```python
from build123d import *

# Parameters (mm, degrees)
SKETCH1_W      = 25.4
SKETCH1_H      = 12.7
SKETCH1_R      = 1.27
EXTRUDE1_DEPTH = 7.62
CHAMFER1_SIZE  = 1.27


with BuildPart() as part:
    # Sketch1 → Extrude1 (new body)
    with BuildSketch(Plane.XY):
        with Locations((12.7, 6.35)):
            Rectangle(SKETCH1_W, SKETCH1_H)
        with Locations((16.51, 6.35)):
            Circle(SKETCH1_R, mode=Mode.SUBTRACT)
    extrude(amount=EXTRUDE1_DEPTH)

    # Chamfer1
    chamfer1_edges = [part.edges().sort_by_distance(p)[0] for p in [
        (0, 6.35, 7.62),
        (0, 6.35, 0),
        (0, 12.7, 3.81),
        (25.4, 12.7, 3.81),
        (25.4, 0, 3.81),
        (0, 0, 3.81),
    ]]
    chamfer(chamfer1_edges, length=CHAMFER1_SIZE)

    # Sketch2 → CBORE for #8 Socket Head Cap Screw1 (revolve, cut)
    with BuildSketch(Plane(origin=(16.51, 6.35, 7.62), x_dir=(0, -1, 0), z_dir=(1, 0, 0))):
        Polygon((0, 0), (0, 7.62), (2.8829, 7.62), (2.2479, 6.985), (2.2479, 4.8006), (2.8829, 4.1656), (3.96875, 4.1656), (3.96875, 0.635), (4.60375, 0), align=None)
    revolve(axis=Axis((16.51, 6.35, 13.97), (0, 0, -1)), mode=Mode.SUBTRACT)

    # Sketch4 → CBORE for #4 Socket Head Cap Screw1 (revolve, cut)
    with BuildSketch(Plane(origin=(3.81, 6.35, 0), x_dir=(0, 1, 0), z_dir=(1, 0, 0))):
        Polygon((0, 0), (0, 7.62), (1.5875, 7.62), (1.5875, 1.524), (1.6002, 1.524), (1.6002, 0.3048), (1.905, 0), align=None)
    revolve(axis=Axis((3.81, 6.35, -6.35), (0, 0, 1)), mode=Mode.SUBTRACT)


solid = part.part
```
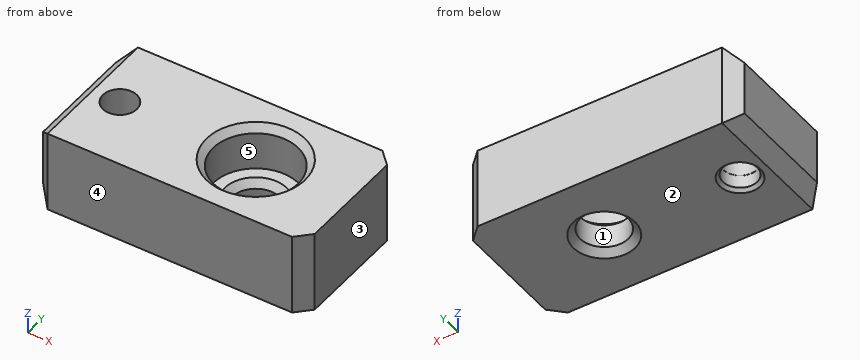
Source: CAD feature listing. Evaluate the final solid. Frame: model axes, mm. Face numbers are marked on the shaded views. A direction names the side the tool comes from. Give positions to 0.01 mm unless a question says otherwise; leave off trailing zeros. Order: outer loops, then holes, each group sorted by start corner. A loop starts at its lowest first (then second) coordinate and runs counter-clockwise, first axis right, second up.
(1) Material intervals for line 1 along X through (y, z) = (6.35, 4.9); line 2 along X through (y, z) = (6.35, 2.1); line 3 along Y through (x, z) = (3.81, 5), sorted ascending.
(2) Section query A-A (y = 6.35). State how many separate pieces and enclosed holes the cut face has, plus the area to 3 significant figures.
(3) Contact query for flat-ended pins moving along their axis: P1, Ø5, axis at x = 16.51, y = 6.35, coming from the -Z side; P2, Ø4, axis at x = 17.5, y = 7, coming from the +Z side. Output: stop coordinate, or through.
(4) Pull-direction query (X, two-part tool) for the marked faces 1, 2 and 3; classes: +X half, -X half, draft (parallel to the pull), parting line (faces both ways), or undercut.
(5) Access query for the marked faces 4 and 5. Directions: +Z, -Z, +X, -X, +Y, -Y. A direction counts if a zero-diameter tool reaches every point of the face in a straight line with its end or side. Return the directions, or none.
(6) Section query C-C (x = 16.51). Return the cut outline in (y, z) (3 decimals), plus the area to 3 significant figures.
Outcome:
1. line 1: x = 0 to 2.22, 5.4 to 12.54, 20.48 to 25.4
1. line 2: x = 0 to 2.22, 5.4 to 14.26, 18.76 to 25.4
1. line 3: y = 0 to 4.76, 7.94 to 12.7
2. separate pieces: 3
2. enclosed holes: 0
2. area: 118 mm2
3. P1: stops at z = 0.38
3. P2: stops at z = 3.45
4. face 1: undercut
4. face 2: draft
4. face 3: +X half
5. face 4: +Z, -Z, +X, -X, -Y
5. face 5: +Z
6. outline: (0, 0) - (3.467, 0) - (4.102, 0.635) - (4.102, 2.819) - (3.467, 3.454) - (2.381, 3.454) - (2.381, 6.985) - (1.746, 7.62) - (0, 7.62) - close; (8.598, 0.635) - (9.233, 0) - (12.7, 0) - (12.7, 7.62) - (10.954, 7.62) - (10.319, 6.985) - (10.319, 3.454) - (9.233, 3.454) - (8.598, 2.819) - close
6. area: 47.0 mm2
